```python
from build123d import *

# Parameters (mm, degrees)
F0_R     = 16
F0_R_2   = 13.6
F1_DEPTH = 5
F2_R     = 15
F2_R_2   = 11.6
F3_DEPTH = 25


with BuildPart() as f1:
    # F0 (on Right) → F1 (new body)
    with BuildSketch(Plane.YZ):
        Circle(F0_R)
        Circle(F0_R_2, mode=Mode.SUBTRACT)
    extrude(amount=F1_DEPTH)

    # F2 (on face) → F3 (join)
    with BuildSketch(Plane(origin=(0, 0, 0), x_dir=(0, -1, 0), z_dir=(-1, 0, 0))):
        Circle(F2_R)
        Circle(F2_R_2, mode=Mode.SUBTRACT)
    extrude(amount=F3_DEPTH)


solid = f1.part
```
Here's how the part is built. I have some questions about the finished solid (model axes, mm). A direction names the side the tool comes from. Give positions to 0.01 mm unless a question says otherwise; leave off trailing zeros. Order: outer loops, then holes, each group sorted by start corner. A loop starts at its lowest first (then second) coordinate and runs counter-clockwise, first axis right, second up. Notation, with made-up numbers: (-26, -40) - (33, -40) arc R20 ccw to (33, -12) - close; hole circle Ø6 at (42.25, 22.5). An arc over 180 degrees is marked (long way). Answer as a JSON object with one key per item and string values. Group by question number.
Item 1: If we section it at C-C on x = -0.5: Please give me the cut outline in (y, z).
Item 2: If we section it at A-A on z = 0: Please give me the cut outline in (x, y), and give its area (3 significant figures).
Item 3: Please list where these lines run through material, in increasing order: probe 1 along Z at (x, y) = (2.15, 0); probe 2 along Z at (x, y) = (-13.25, 0); probe 3 along X at (y, z) = (-8.5, 10.5).
Item 4: For P1, Ø1.5, axis at x = -20.5, z = -9, coming from the +Y side; P2, Ø10, axis at x = -19.5, y = 9, coming from the -Z side; P3, Ø3, axis at x = -20.5, y = -4.5, coming from the +Z side; P4, Ø9.5, axis at y = -5.5, z = 1.5, coming from the -X side, each with a flat end and sliding along its axis, tell me the tip position at first contact or that it passes through.
Item 5: Which directions (+Z, -Z, +X, -X, +Y, -Y) give clear straight access to the entire face, cutting with the end or side of a thin tool? Please do faces 4 (the cylindrical face through (2.465, -2.948, -13.277)), 5 (the flat face through (-25, -8, -9)).
Item 6: If we mould it in two halves opening along Z, with no side actions, what happens to faces 1 (the flat face through (0, -11.02, 4.09)), 2 (the cylindrical face through (-12.325, 14.985, 0.66)), 3 (the flat face through (5, -7, -12))? For each: pulls with the +Z half, pulls with the -Z half, needs draft (parallel to the pull), parting line crosses it, or undercut.
Result set:
{
 "1": {"outline": "circle Ø30 at (0, 0); hole circle Ø23.2 at (0, 0)"},
 "2": {"outline": "(-25, -15) - (0, -15) - (0, -16) - (5, -16) - (5, -13.6) - (0, -13.6) - (0, -11.6) - (-25, -11.6) - close; (-25, 11.6) - (0, 11.6) - (0, 13.6) - (5, 13.6) - (5, 16) - (0, 16) - (0, 15) - (-25, 15) - close", "area": "194 mm²"},
 "3": {"probe 1": "-16 to -13.6, 13.6 to 16", "probe 2": "-15 to -11.6, 11.6 to 15", "probe 3": "-25 to 0"},
 "4": {"P1": "y = 12.53", "P2": "z = -14.46", "P3": "z = 14.7", "P4": "through"},
 "5": {"face 4": "+X", "face 5": "+Z, -Z, -X, +Y, -Y"},
 "6": {"face 1": "undercut", "face 2": "parting line crosses it", "face 3": "needs draft"}
}
